Build history of the part. All positions in model axes, mm. Face numbers are marked on the shaded views. A direction names the side the tool comes from. Round coordinates to 2 decimals unless told otherwise and drop trailing zeros. Write each loop counter-clockwise with the first axis right and the second up, starting at its lowest first coordinate (ties: lowest second). Pieces come first, ordered by that corner, then holes. Notation, with made-up numbers: (84.25, 44) -> (129.25, 44) arc R28 cw to (129.25, 76) -> close; hole circle Ø3 at (16, -3). An arc over 180 degrees is marked (long way). Answer in a Markdown table with one row per item. Add a question column.
from build123d import *

# Parameters (mm, degrees)
F1_DEPTH      = 120.65
F2_W          = 114.3
F2_H          = 139.7
F2_W_2        = 63.5
F2_H_2        = 63.5
F3_DEPTH      = 139.7
F4_DEPTH      = 165.1
F5_DEPTH      = 271.526
F5_DEPTH_BACK = 305.054
F6_DEPTH      = 87.122
F7_DEPTH      = 165.1
F8_R          = 25.4
F9_DEPTH      = 72.39


with BuildPart() as f1:
    # F0 (on Front) → F1 (new body, symmetric)
    with BuildSketch(Plane.XZ):
        Polygon((-101.9933745265, 279.4), (-101.9933745265, 0), (101.2066254735, 0), align=None)
        Polygon((-101.9933745265, 279.4), (101.2066254735, 0), (101.2066254735, 279.4), align=None)
    extrude(amount=F1_DEPTH, both=True)

    # F2 (on face) → F3 (cut)
    with BuildSketch(Plane.YZ.offset(101.2066254735)):
        with Locations((0, 146.05)):
            Rectangle(F2_W, F2_H)
        with Locations((0, 158.75)):
            Rectangle(F2_W_2, F2_H_2, mode=Mode.SUBTRACT)
        with Locations((0, 158.75)):
            Rectangle(F2_W_2, F2_H_2)
    extrude(amount=-F3_DEPTH, mode=Mode.SUBTRACT)

    # F2 (on face) → F4 (join)
    with BuildSketch(Plane.YZ.offset(101.2066254735)):
        with Locations((0, 158.75)):
            Rectangle(F2_W_2, F2_H_2)
    extrude(amount=-F4_DEPTH)

    # F0 (on Front) → F5 (cut, two sides)
    with BuildSketch(Plane.XZ) as f5_sk:
        Polygon((-101.9933745265, 279.4), (101.2066254735, 0), (101.2066254735, 279.4), align=None)
    extrude(amount=F5_DEPTH, mode=Mode.SUBTRACT)
    extrude(f5_sk.sketch, amount=-F5_DEPTH_BACK, mode=Mode.SUBTRACT)

    # F6 (cut): a face of the model
    f6_faces = [f1.faces().sort_by_distance(p)[0] for p in [
        (-22.7054235885, -31.75, 148.6706349206),
    ]]
    extrude(f6_faces, amount=-F6_DEPTH, mode=Mode.SUBTRACT)

    # F2 (on face) → F7 (cut)
    with BuildSketch(Plane.YZ.offset(101.2066254735)):
        with Locations((0, 158.75)):
            Rectangle(F2_W_2, F2_H_2)
    extrude(amount=-F7_DEPTH, mode=Mode.SUBTRACT)

    # F8 (on face) → F9 (cut)
    with BuildSketch(Plane.XY.offset(76.2)):
        Circle(F8_R)
    extrude(amount=-F9_DEPTH, mode=Mode.SUBTRACT)


solid = f1.part
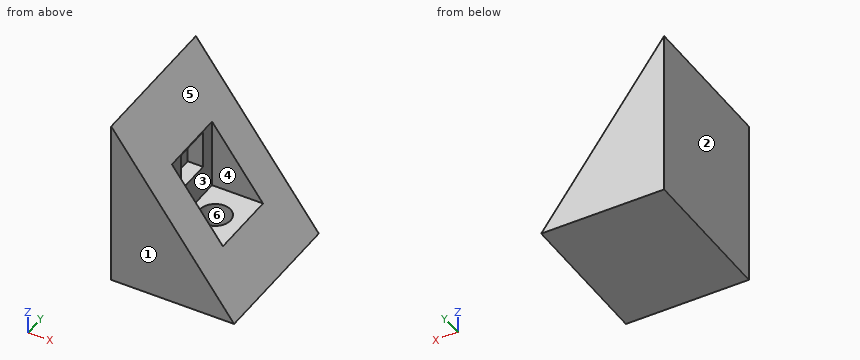
(1) Saw through at A-A (y = 0). List the corners of the cut face in (x, z), plus the area to 3 significant figures.
(2) Mould opens along Y. For the marked faces 1, 2 and 3 say: pulls with the +Y half, pulls with the -Y half, needs draft (parallel to the pull), parting line crosses it, or undercut.
(3) Saw through at B-B (z = 23). List the corners of the cut face in (x, y), plus the area to 3 significant figures.
(4) Which spindle directions (+Z, -Z, +X, -X, +Y, -Y) get a long thin tool onto all of the face, cutting with end or side? Do the marked faces 4, 5 and 6. Say none if no direction does.
(5) Saw through at D-D (x = -55). List the corners of the cut face in (y, z), plus the area to 3 significant figures.
(6) Probe line 1 along Y through (x, z) = (-36.5, 86); line 2 along Y through (x, z) = (0, 46.5); line 3 along Z through (x, y) = (14.5, 23). List the from-to ranges inside material, lowest first.
(7) Drop flat-ended pins along their axis: P1, Ø10, axis at y = -44, z = 32, coming from the +X side; P2, Ø3, axis at y = 13, z = 62, coming from the +X side; P3, Ø8, axis at y = -16.5, z = 61, coming from the +X side. Give the stop position or say it passes through.
(8) Saw through at C-C (x = 9.5). List the corners of the cut face in (y, z), plus the area to 3 significant figures.
Answer sheet:
| question | item | result |
|---|---|---|
| 1 | outline | (-101.99, 0) -> (101.21, 0) -> (45.79, 76.2) -> (25.4, 76.2) -> (25.4, 3.81) -> (-25.4, 3.81) -> (-25.4, 76.2) -> (-38.49, 76.2) -> (-38.49, 127) -> (-63.89, 127) -> (-63.89, 190.5) -> (-38.49, 190.5) -> (-38.49, 192.09) -> (-101.99, 279.4) -> close |
| 1 | area | 18,200 mm² |
| 2 | face 1 | pulls with the -Y half |
| 2 | face 2 | needs draft |
| 2 | face 3 | undercut |
| 3 | outline | (-101.99, -120.65) -> (84.48, -120.65) -> (84.48, 120.65) -> (-101.99, 120.65) -> close; hole circle Ø50.8 at (0, 0) |
| 3 | area | 43,000 mm² |
| 4 | face 4 | +Z, +X |
| 4 | face 5 | +Z, +X, +Y, -Y |
| 4 | face 6 | +Z |
| 5 | outline | (-120.65, 0) -> (120.65, 0) -> (120.65, 214.78) -> (-120.65, 214.78) -> close; hole (-31.75, 127) -> (31.75, 127) -> (31.75, 190.5) -> (-31.75, 190.5) -> close |
| 5 | area | 47,800 mm² |
| 6 | line 1 | y = -120.65 to -57.15, 57.15 to 120.65 |
| 6 | line 2 | y = -120.65 to -25.4, 25.4 to 120.65 |
| 6 | line 3 | z = 0 to 76.2 |
| 7 | P1 | stops at x = 81.57 |
| 7 | P2 | stops at x = 57.21 |
| 7 | P3 | stops at x = 59.75 |
| 8 | outline | (-120.65, 0) -> (120.65, 0) -> (120.65, 126.1) -> (57.15, 126.1) -> (57.15, 76.2) -> (23.56, 76.2) -> (23.56, 3.81) -> (-23.56, 3.81) -> (-23.56, 76.2) -> (-57.15, 76.2) -> (-57.15, 126.1) -> (-120.65, 126.1) -> close |
| 8 | area | 21,300 mm² |
